The model under review builds one solid part; all positions refer to its coordinate system, in mm. A direction names the side the tool comes from. Round coordinates to 2 decimals unless told otherwise and drop trailing zeros. Loops run counter-clockwise (first coordinate to the right, second up) from the corner with the lowest first, then second, coordinate; pieces in that order, holes last. Notation, with made-up numbers: (42.25, 35.5) -> (76.25, 35.5) arc R21 cw to (76.25, 44.5) -> close; hole circle Ø1 at (4.5, 23.5). An arc over 180 degrees is marked (long way). Write each question's results on one line, items separated by ' | '. Start each with the question number.
Item 1: We need section A-A (x = 0). Give the boundary of the cut face in (y, z).
Item 2: For L1, parallel to Y at x = 0, z = -4.6; L2, parallel to Y at x = 40, z = -5.85; L3, parallel to X at y = 8, z = -6.25, list the stretches that pass through material, from the lowest coordinate up. Write a range as from..to.
Item 3: Mouldability with a two-part tool opening along Y and no side actions: class faces 4 (the flat face through (-0.035, -45.889, -15.285)), 5 (the flat face through (-33, 60, -8)), 6 (the cylindrical face through (0.59, 84.46, -5.54)) as pulls with the +Y half, pulls with the -Y half, needs draft (parallel to the pull), parting line crosses it, or undercut.
Item 4: We need section C-C (y = 40). Give the boundary of the cut face in (x, z).
Item 5: We need section B-B (z = -13.5). Give the boundary of the cut face in (x, y), and give its area (3 significant figures).
Item 6: Tool access review of faces 1 (the cylindrical face through (53.07, -48.66, -1.52)), 2 (the flat face through (2.5, 39, -11)), 3 (the flat face through (-0.035, 45.889, -15.285)): name each direction out of +Z, -Z, +X, -X, +Y, -Y from which nothing blocks a thin tool from reaching the whole face with its end or side.
Item 7: Clearance check with flat-ended pins moving along their axes: pin 1 Ø14.5 at (x, y) = (40, -69.28) entering from -Z; pin 2 Ø2 at (x, y) = (48.5, 12) entering from -Z; pin 3 Ø5 at (x, z) = (-50.5, -14) entering from -Y. State where each tip first meets the part, or that it passes through.
from build123d import *

# Parameters (mm, degrees)
IZIM2_R               = 20
KES_EKSTR_ZYON1_DEPTH = 130.340635533
FEDER6_REACH          = 131.341
IZIM3_WALL_W          = 307.641360504
IZIM3_WALL_H          = 5
FEDER7_REACH          = 131.341
IZIM4_WALL_W          = 307.641360504
IZIM4_WALL_H          = 5
KES_EKSTR_ZYON2_REACH = 130.16
IZIM5_R               = 4.5


with BuildPart() as part:
    # Çizim1 → Döndür1 (revolve)
    with BuildSketch(Plane(origin=(0, 0, 0), x_dir=(0, 0, -1), z_dir=(1, 0, 0)), mode=Mode.PRIVATE) as d_nd_r1_sk:
        Polygon((0, 20), (0, 72), (3, 72), (3, 90), (8, 90), (8, 67.5), (5, 67.5), (5, 25), (23, 25), (23, 0), (0, 0), align=None)
    revolve(d_nd_r1_sk.sketch.rotate(Axis((0, 0, 0), (0, 0, 1)), 90), axis=Axis((0, 0, 0), (0, 0, 1)))

    # Çizim2 → Kes-Ekstrüzyon1 (cut, through all)
    with BuildSketch(Plane(origin=(0, 0, -23), x_dir=(-1, 0, 0), z_dir=(0, 0, -1))):
        Circle(IZIM2_R)
    extrude(amount=-KES_EKSTR_ZYON1_DEPTH, mode=Mode.SUBTRACT)

    # Çizim3 wall → Feder6 (add, up to next)
    with BuildSketch(Plane(origin=(0, 45.25, -15.5), x_dir=(0, 0.947613186704, 0.319420175294), z_dir=(0, -0.319420175294, 0.947613186704)), mode=Mode.PRIVATE) as feder6_sk1:
        Rectangle(IZIM3_WALL_W, IZIM3_WALL_H)
    feder6_tool1 = extrude(feder6_sk1.sketch, amount=FEDER6_REACH, mode=Mode.PRIVATE) - part.part
    feder6 = feder6_tool1.solids().sort_by_distance((0, 45.25, -15.5))[0]
    add(feder6)

    # Aynalama1: Feder6 across plane
    add(feder6.mirror(Plane.ZX))

    # Çizim4 wall → Feder7 (add, up to next)
    with BuildSketch(Plane(origin=(-45.25, 0, -15.5), x_dir=(-0.947613186704, 0, 0.319420175294), z_dir=(0.319420175294, 0, 0.947613186704)), mode=Mode.PRIVATE) as feder7_sk1:
        Rectangle(IZIM4_WALL_W, IZIM4_WALL_H)
    feder7_tool1 = extrude(feder7_sk1.sketch, amount=FEDER7_REACH, mode=Mode.PRIVATE) - part.part
    feder7 = feder7_tool1.solids().sort_by_distance((-45.25, 0, -15.5))[0]
    add(feder7)

    # Aynalama2: Feder7 across plane
    add(feder7.mirror(Plane(origin=(0, 0, 0), x_dir=(0, 0, 1), z_dir=(1, 0, 0))))

    # Çizim5 → Kes-Ekstrüzyon2 (cut, up to next)
    with BuildSketch(Plane(origin=(0, 0, -8), x_dir=(-1, 0, 0), z_dir=(0, 0, -1)), mode=Mode.PRIVATE) as kes_ekstr_zyon2_sk1:
        with Locations((0, 80)):
            Circle(IZIM5_R)
    kes_ekstr_zyon2_tool1 = extrude(kes_ekstr_zyon2_sk1.sketch, amount=-KES_EKSTR_ZYON2_REACH, mode=Mode.PRIVATE) & part.part
    # Çizim5 → Kes-Ekstrüzyon2 (cut, up to next)
    with BuildSketch(Plane(origin=(0, 0, -8), x_dir=(-1, 0, 0), z_dir=(0, 0, -1)), mode=Mode.PRIVATE) as kes_ekstr_zyon2_sk2:
        with Locations((40, 69.282032303)):
            Circle(IZIM5_R)
    kes_ekstr_zyon2_tool2 = extrude(kes_ekstr_zyon2_sk2.sketch, amount=-KES_EKSTR_ZYON2_REACH, mode=Mode.PRIVATE) & part.part
    # Çizim5 → Kes-Ekstrüzyon2 (cut, up to next)
    with BuildSketch(Plane(origin=(0, 0, -8), x_dir=(-1, 0, 0), z_dir=(0, 0, -1)), mode=Mode.PRIVATE) as kes_ekstr_zyon2_sk3:
        with Locations((69.282032303, 40)):
            Circle(IZIM5_R)
    kes_ekstr_zyon2_tool3 = extrude(kes_ekstr_zyon2_sk3.sketch, amount=-KES_EKSTR_ZYON2_REACH, mode=Mode.PRIVATE) & part.part
    # Çizim5 → Kes-Ekstrüzyon2 (cut, up to next)
    with BuildSketch(Plane(origin=(0, 0, -8), x_dir=(-1, 0, 0), z_dir=(0, 0, -1)), mode=Mode.PRIVATE) as kes_ekstr_zyon2_sk4:
        with Locations((80, 0)):
            Circle(IZIM5_R)
    kes_ekstr_zyon2_tool4 = extrude(kes_ekstr_zyon2_sk4.sketch, amount=-KES_EKSTR_ZYON2_REACH, mode=Mode.PRIVATE) & part.part
    # Çizim5 → Kes-Ekstrüzyon2 (cut, up to next)
    with BuildSketch(Plane(origin=(0, 0, -8), x_dir=(-1, 0, 0), z_dir=(0, 0, -1)), mode=Mode.PRIVATE) as kes_ekstr_zyon2_sk5:
        with Locations((69.282032303, -40)):
            Circle(IZIM5_R)
    kes_ekstr_zyon2_tool5 = extrude(kes_ekstr_zyon2_sk5.sketch, amount=-KES_EKSTR_ZYON2_REACH, mode=Mode.PRIVATE) & part.part
    # Çizim5 → Kes-Ekstrüzyon2 (cut, up to next)
    with BuildSketch(Plane(origin=(0, 0, -8), x_dir=(-1, 0, 0), z_dir=(0, 0, -1)), mode=Mode.PRIVATE) as kes_ekstr_zyon2_sk6:
        with Locations((40, -69.282032303)):
            Circle(IZIM5_R)
    kes_ekstr_zyon2_tool6 = extrude(kes_ekstr_zyon2_sk6.sketch, amount=-KES_EKSTR_ZYON2_REACH, mode=Mode.PRIVATE) & part.part
    # Çizim5 → Kes-Ekstrüzyon2 (cut, up to next)
    with BuildSketch(Plane(origin=(0, 0, -8), x_dir=(-1, 0, 0), z_dir=(0, 0, -1)), mode=Mode.PRIVATE) as kes_ekstr_zyon2_sk7:
        with Locations((0, -80)):
            Circle(IZIM5_R)
    kes_ekstr_zyon2_tool7 = extrude(kes_ekstr_zyon2_sk7.sketch, amount=-KES_EKSTR_ZYON2_REACH, mode=Mode.PRIVATE) & part.part
    # Çizim5 → Kes-Ekstrüzyon2 (cut, up to next)
    with BuildSketch(Plane(origin=(0, 0, -8), x_dir=(-1, 0, 0), z_dir=(0, 0, -1)), mode=Mode.PRIVATE) as kes_ekstr_zyon2_sk8:
        with Locations((-40, -69.282032303)):
            Circle(IZIM5_R)
    kes_ekstr_zyon2_tool8 = extrude(kes_ekstr_zyon2_sk8.sketch, amount=-KES_EKSTR_ZYON2_REACH, mode=Mode.PRIVATE) & part.part
    # Çizim5 → Kes-Ekstrüzyon2 (cut, up to next)
    with BuildSketch(Plane(origin=(0, 0, -8), x_dir=(-1, 0, 0), z_dir=(0, 0, -1)), mode=Mode.PRIVATE) as kes_ekstr_zyon2_sk9:
        with Locations((-69.282032303, -40)):
            Circle(IZIM5_R)
    kes_ekstr_zyon2_tool9 = extrude(kes_ekstr_zyon2_sk9.sketch, amount=-KES_EKSTR_ZYON2_REACH, mode=Mode.PRIVATE) & part.part
    # Çizim5 → Kes-Ekstrüzyon2 (cut, up to next)
    with BuildSketch(Plane(origin=(0, 0, -8), x_dir=(-1, 0, 0), z_dir=(0, 0, -1)), mode=Mode.PRIVATE) as kes_ekstr_zyon2_sk10:
        with Locations((-80, 0)):
            Circle(IZIM5_R)
    kes_ekstr_zyon2_tool10 = extrude(kes_ekstr_zyon2_sk10.sketch, amount=-KES_EKSTR_ZYON2_REACH, mode=Mode.PRIVATE) & part.part
    # Çizim5 → Kes-Ekstrüzyon2 (cut, up to next)
    with BuildSketch(Plane(origin=(0, 0, -8), x_dir=(-1, 0, 0), z_dir=(0, 0, -1)), mode=Mode.PRIVATE) as kes_ekstr_zyon2_sk11:
        with Locations((-69.282032303, 40)):
            Circle(IZIM5_R)
    kes_ekstr_zyon2_tool11 = extrude(kes_ekstr_zyon2_sk11.sketch, amount=-KES_EKSTR_ZYON2_REACH, mode=Mode.PRIVATE) & part.part
    # Çizim5 → Kes-Ekstrüzyon2 (cut, up to next)
    with BuildSketch(Plane(origin=(0, 0, -8), x_dir=(-1, 0, 0), z_dir=(0, 0, -1)), mode=Mode.PRIVATE) as kes_ekstr_zyon2_sk12:
        with Locations((-40, 69.282032303)):
            Circle(IZIM5_R)
    kes_ekstr_zyon2_tool12 = extrude(kes_ekstr_zyon2_sk12.sketch, amount=-KES_EKSTR_ZYON2_REACH, mode=Mode.PRIVATE) & part.part
    add(kes_ekstr_zyon2_tool1.solids().sort_by_distance((0, 80, -8))[0], mode=Mode.SUBTRACT)
    add(kes_ekstr_zyon2_tool2.solids().sort_by_distance((-40, 69.282032, -8))[0], mode=Mode.SUBTRACT)
    add(kes_ekstr_zyon2_tool3.solids().sort_by_distance((-69.282032, 40, -8))[0], mode=Mode.SUBTRACT)
    add(kes_ekstr_zyon2_tool4.solids().sort_by_distance((-80, 0, -8))[0], mode=Mode.SUBTRACT)
    add(kes_ekstr_zyon2_tool5.solids().sort_by_distance((-69.282032, -40, -8))[0], mode=Mode.SUBTRACT)
    add(kes_ekstr_zyon2_tool6.solids().sort_by_distance((-40, -69.282032, -8))[0], mode=Mode.SUBTRACT)
    add(kes_ekstr_zyon2_tool7.solids().sort_by_distance((0, -80, -8))[0], mode=Mode.SUBTRACT)
    add(kes_ekstr_zyon2_tool8.solids().sort_by_distance((40, -69.282032, -8))[0], mode=Mode.SUBTRACT)
    add(kes_ekstr_zyon2_tool9.solids().sort_by_distance((69.282032, -40, -8))[0], mode=Mode.SUBTRACT)
    add(kes_ekstr_zyon2_tool10.solids().sort_by_distance((80, 0, -8))[0], mode=Mode.SUBTRACT)
    add(kes_ekstr_zyon2_tool11.solids().sort_by_distance((69.282032, 40, -8))[0], mode=Mode.SUBTRACT)
    add(kes_ekstr_zyon2_tool12.solids().sort_by_distance((40, 69.282032, -8))[0], mode=Mode.SUBTRACT)


solid = part.part
Here are the results:
1) outline: (-90, -8) -> (-84.5, -8) -> (-84.5, -3) -> (-90, -3) -> close; (-75.5, -8) -> (-67.5, -8) -> (-25, -22.33) -> (-25, -23) -> (-20, -23) -> (-20, 0) -> (-72, 0) -> (-72, -3) -> (-75.5, -3) -> close; (20, -23) -> (25, -23) -> (25, -22.33) -> (67.5, -8) -> (75.5, -8) -> (75.5, -3) -> (72, -3) -> (72, 0) -> (20, 0) -> close; (84.5, -8) -> (90, -8) -> (90, -3) -> (84.5, -3) -> close
2) L1: y = -90..-84.5, -75.5..-20, 20..75.5, 84.5..90 | L2: y = -80.62..-73.78, -64.78..-54.37, -2.5..2.5, 54.37..64.78, 73.78..80.62 | L3: x = -89.64..-67.02, -23.69..-18.33, 18.33..23.69, 67.02..89.64
3) face 4: pulls with the -Y half | face 5: needs draft | face 6: undercut
4) outline: (-80.62, -8) -> (-73.78, -8) -> (-73.78, -3) -> (-80.62, -3) -> close; (-64.78, -8) -> (-54.37, -8) -> (-54.37, -5) -> (-2.5, -5) -> (-2.5, -17.27) -> (2.5, -17.27) -> (2.5, -5) -> (54.37, -5) -> (54.37, -8) -> (64.78, -8) -> (64.78, -3) -> (59.87, -3) -> (59.87, 0) -> (-59.87, 0) -> (-59.87, -3) -> (-64.78, -3) -> close; (73.78, -8) -> (80.62, -8) -> (80.62, -3) -> (73.78, -3) -> close
5) outline: (-51.18, -2.5) -> (-24.87, -2.5) arc R25 ccw to (-2.5, -24.87) -> (-2.5, -51.18) -> (2.5, -51.18) -> (2.5, -24.87) arc R25 ccw to (24.87, -2.5) -> (51.18, -2.5) -> (51.18, 2.5) -> (24.87, 2.5) arc R25 ccw to (2.5, 24.87) -> (2.5, 51.18) -> (-2.5, 51.18) -> (-2.5, 24.87) arc R25 ccw to (-24.87, 2.5) -> (-51.18, 2.5) -> close; hole circle Ø40 at (0, 0) | area: 1,230 mm2
6) face 1: +Z | face 2: -Z | face 3: -Z, +X, -X, +Y
7) pin 1: stops at z = -8 | pin 2: stops at z = -5 | pin 3: stops at y = -2.5
